Work out the finished part from the listing and answer in its coordinate system (mm). A direction names the side the tool comes from. Coordinates: 2 decimals unless noted, no trailing zeros. Order: outer loops, then holes, each group sorted by start corner. A loop starts at its lowest first (then second) coordinate and runs counter-clockwise, first axis right, second up.
```python
from build123d import *

# Parameters (mm, degrees)
SKETCH2_W                 = 27
SKETCH2_H                 = 40
BOSS_EXTRUDE1_DEPTH       = 2.5
SKETCH3_W                 = 27
SKETCH3_H                 = 40
SKETCH3_W_2               = 24
SKETCH3_H_2               = 37
BOSS_EXTRUDE2_DEPTH       = 12
BOSS_EXTRUDE3_DEPTH       = 4
SKETCH5_W                 = 7.3
SKETCH5_H                 = 7.3
BOSS_EXTRUDE4_DEPTH       = 3
F_3_0MM_DOWEL_HOLE1_D     = 3.1
F_3_0MM_DOWEL_HOLE1_DEPTH = 2.8
F_3_0MM_DOWEL_HOLE1_TIP   = 0.931333959
REVOLVE1_ANGLE            = 180
MIRROR2_COPY_1_DEPTH      = 4
MIRROR2_COPY_2_ANGLE      = 180
FILLET1_R                 = 1


with BuildPart() as part:
    # Sketch2 → Boss-Extrude1 (new body)
    with BuildSketch(Plane(origin=(0, 0, 0), x_dir=(1, 0, 0), z_dir=(0, 1, 0))):
        Rectangle(SKETCH2_W, SKETCH2_H)
    extrude(amount=BOSS_EXTRUDE1_DEPTH)

    # Sketch3 → Boss-Extrude2 (add)
    with BuildSketch(Plane(origin=(0, 2.5, 0), x_dir=(1, 0, 0), z_dir=(0, 1, 0))):
        Rectangle(SKETCH3_W, SKETCH3_H)
        Rectangle(SKETCH3_W_2, SKETCH3_H_2, mode=Mode.SUBTRACT)
    extrude(amount=BOSS_EXTRUDE2_DEPTH)

    # Sketch4 → Boss-Extrude3 (add)
    with BuildSketch(Plane.XY.offset(20)):
        with BuildLine():
            Line((15.5, 14.5), (13.5, 14.5))
            Line((13.5, 14.5), (13.5, 11.5))
            Line((13.5, 11.5), (18.5, 11.5))
            ThreePointArc((18.5, 11.5), (20.621320344, 16.621320344), (15.5, 14.5))
        make_face()
    boss_extrude3 = extrude(amount=-BOSS_EXTRUDE3_DEPTH)

    # Sketch5 → Boss-Extrude4 (add)
    with BuildSketch(Plane(origin=(0, 2.5, 0), x_dir=(1, 0, 0), z_dir=(0, 1, 0))):
        with Locations((-6.35, 10.16)):
            Rectangle(SKETCH5_W, SKETCH5_H)
        with Locations((6.35, 10.16)):
            Rectangle(SKETCH5_W, SKETCH5_H)
        with Locations((6.35, -10.16)):
            Rectangle(SKETCH5_W, SKETCH5_H)
        with Locations((-6.35, -10.16)):
            Rectangle(SKETCH5_W, SKETCH5_H)
    extrude(amount=BOSS_EXTRUDE4_DEPTH)

    # Ø3.0mm Dowel Hole1
    with Locations(Plane(origin=(0, 5.5, 0), x_dir=(1, 0, 0), z_dir=(0, 1, 0))):
        with Locations((-6.35, 10.16), (6.35, 10.16), (6.35, -10.16), (-6.35, -10.16)):
            Hole(F_3_0MM_DOWEL_HOLE1_D / 2, depth=F_3_0MM_DOWEL_HOLE1_DEPTH)
            with Locations((0, 0, -(F_3_0MM_DOWEL_HOLE1_DEPTH + F_3_0MM_DOWEL_HOLE1_TIP / 2))):  # 118° drill point
                Cone(0, F_3_0MM_DOWEL_HOLE1_D / 2, F_3_0MM_DOWEL_HOLE1_TIP, mode=Mode.SUBTRACT)

    # Sketch13 → Revolve1 (revolve)
    with BuildSketch(Plane(origin=(0, 0, 16), x_dir=(-1, 0, 0), z_dir=(0, 0, -1))):
        with BuildLine():
            Line((-18.5, 16.25), (-18.5, 12.75))
            ThreePointArc((-18.5, 12.75), (-16.75, 14.5), (-18.5, 16.25))
        make_face()
    revolve1 = revolve(axis=Axis((18.5, 11.5, 16), (0, -1, 0)), revolution_arc=REVOLVE1_ANGLE)

    # Mirror1: Boss-Extrude3, Revolve1 across plane
    add(boss_extrude3.mirror(Plane(origin=(0, 0, 12.5), x_dir=(1, 0, 0), z_dir=(0, 0, -1))))
    add(revolve1.mirror(Plane(origin=(0, 0, 12.5), x_dir=(1, 0, 0), z_dir=(0, 0, -1))))

    # Mirror2: Boss-Extrude3, Revolve1 across plane
    add(boss_extrude3.mirror(Plane(origin=(0, 0, 0), x_dir=(1, 0, 0), z_dir=(0, 0, -1))))
    add(revolve1.mirror(Plane(origin=(0, 0, 0), x_dir=(1, 0, 0), z_dir=(0, 0, -1))))

    # Mirror2 copy 1 sketch → Mirror2 copy 1 (add)
    with BuildSketch(Plane.XY.offset(-5)):
        with BuildLine():
            Line((15.5, 14.5), (13.5, 14.5))
            Line((13.5, 14.5), (13.5, 11.5))
            Line((13.5, 11.5), (18.5, 11.5))
            ThreePointArc((18.5, 11.5), (20.621320344, 16.621320344), (15.5, 14.5))
        make_face()
    extrude(amount=-MIRROR2_COPY_1_DEPTH)

    # Mirror2 copy 2 sketch → Mirror2 copy 2 (revolve)
    with BuildSketch(Plane(origin=(0, 0, -9), x_dir=(-1, 0, 0), z_dir=(0, 0, -1))):
        with BuildLine():
            Line((-18.5, 16.25), (-18.5, 12.75))
            ThreePointArc((-18.5, 12.75), (-16.75, 14.5), (-18.5, 16.25))
        make_face()
    revolve(axis=Axis((18.5, 11.5, -9), (0, -1, 0)), revolution_arc=MIRROR2_COPY_2_ANGLE)

    # Fillet1
    fillet1_edges = [part.edges().sort_by_distance(p)[0] for p in [
        (13.5, 5.75, -20),
        (13.5, 5.75, 20),
        (0, 0, 20),
        (-13.5, 0, 0),
        (0, 0, -20),
        (13.5, 0, 0),
        (-13.5, 7.25, 20),
        (-13.5, 7.25, -20),
    ]]
    fillet(fillet1_edges, radius=FILLET1_R)


solid = part.part
```
1. For faces 1 (the flat face through (2.7, 4, 10)), 2 (the flat face through (13, 14.5, 0)), 3 (the cylindrical face through (0.175, 0.301, -19.715)), determine the directions among +Z, -Z, +X, -X, +Y, -Y from which every point of the face is accessible in a straight line to the end or side of a thin tool.
2. The part is cut by section D-D (z = 7). Determine the outline of the cut face in (x, y).
3. The part is cut by section A-A (x = 14). Determine the outline of the cut face in (y, z), plus the area to 3 significant figures.
4. The part is cut by section B-B (z = -1.5). Determine the outline of the cut face in (x, y).
5. The part is cut by section C-C (y = 7.75). Determine the outline of the cut face in (x, z), plus the area to 3 significant figures.
6. Flat-ended cylindrical pins translate along their axes: pin 1 (4 mm diameter, centred on x = -6.35, z = -10.16, fed in from +Y); pin 2 (3.5 mm diameter, centred on y = 3.5, z = -8.5, fed in from +X); pin 3 (3 mm diameter, centred on y = 15.5, z = 14, fed in from +X). Find the tip coordinate at first contact, or state that the pin passes through.
7. The mould has two halves that part along Z. Classify faces 4 (the flat face through (6, 5.5, 12)), 5 (the flat face through (16, 11.5, -18)), 6 (the cylindrical face through (13.215, 6.176, -19.699)): released by +Z, released by -Z, zero draft, split by the parting line, or undercut.
8. Consider probe 1 along X at (y, z) = (4.2, 10.16); probe 2 along Z at (x, y) = (-6.35, 4); probe 3 along X at (y, z) = (8, 11). Determine where each line is inside the solid, lowest interval first.
Worked out:
1. face 1: +Y
1. face 2: +Z, -Z, -X, +Y
1. face 3: -Z, +X, -X, -Y
2. outline: (-13.5, 1) arc R1 ccw to (-12.5, 0) - (12.5, 0) arc R1 ccw to (13.5, 1) - (13.5, 11.5) - (18.5, 11.5) arc R3 ccw (long way) to (15.5, 14.5) - (12, 14.5) - (12, 2.5) - (10, 2.5) - (10, 5.5) - (2.7, 5.5) - (2.7, 2.5) - (-2.7, 2.5) - (-2.7, 5.5) - (-10, 5.5) - (-10, 2.5) - (-12, 2.5) - (-12, 14.5) - (-13.5, 14.5) - close
3. outline: (11.5, -20) - (14.5, -20) - (14.5, -16) - (11.5, -16) - close; (11.5, -9) - (14.5, -9) - (14.5, -5) - (11.5, -5) - close; (11.5, 5) - (14.5, 5) - (14.5, 9) - (11.5, 9) - close; (11.5, 16) - (14.5, 16) - (14.5, 20) - (11.5, 20) - close
3. area: 48.0 mm2
4. outline: (-13.5, 1) arc R1 ccw to (-12.5, 0) - (12.5, 0) arc R1 ccw to (13.5, 1) - (13.5, 14.5) - (12, 14.5) - (12, 2.5) - (-12, 2.5) - (-12, 14.5) - (-13.5, 14.5) - close
5. outline: (-13.5, -19) arc R1 ccw to (-12.5, -20) - (12.5, -20) arc R1 ccw to (13.5, -19) - (13.5, 19) arc R1 ccw to (12.5, 20) - (-12.5, 20) arc R1 ccw to (-13.5, 19) - close; hole (-12, -18.5) - (12, -18.5) - (12, 18.5) - (-12, 18.5) - close
5. area: 191 mm2
6. pin 1: stops at y = 5.5
6. pin 2: stops at x = 13.5
6. pin 3: stops at x = 20.09
7. face 4: undercut
7. face 5: zero draft
7. face 6: released by -Z
8. probe 1: x = -13.5 to -12, -10 to -7.9, -4.8 to -2.7, 2.7 to 4.8, 7.9 to 10, 12 to 13.5
8. probe 2: z = -20 to -18.5, -13.81 to -11.71, -8.61 to -6.51, 6.51 to 8.61, 11.71 to 13.81, 18.5 to 20
8. probe 3: x = -13.5 to -12, 12 to 13.5
